Check sheet for the modelled part. Datum: model origin and axes. Units: mm. A direction names the side the tool comes from. Round coordinates to 2 decimals unless told otherwise and drop trailing zeros. Write each loop counter-clockwise with the first axis right and the second up, starting at its lowest first coordinate (ties: lowest second). Pieces come first, ordered by that corner, then holes. Notation, with made-up numbers: M 32,-17 L 50,-17 A24 cw 50,15 Z; hole C 36,34 d5. An arc over 180 degrees is marked long. One line per item, written item: value.
from build123d import *

# Parameters (mm, degrees)
AUFSATZ_LINEAR_AUSTRAGEN1_DEPTH = 20
SKIZZE2_R                       = 3
SCHNITT_LINEAR_AUSTRAGEN1_DEPTH = 20
SKIZZE3_R                       = 5.25
SCHNITT_LINEAR_AUSTRAGEN2_DEPTH = 6.2
SKIZZE4_R                       = 2.3
SCHNITT_LINEAR_AUSTRAGEN3_DEPTH = 10
VERRUNDUNG1_R                   = 2
FASE1_SIZE                      = 0.5


with BuildPart() as part:
    # Skizze1 → Aufsatz-Linear austragen1 (new body)
    with BuildSketch(Plane.XY):
        Polygon((0, -22.130332374), (0, 22.130332374), (7, 22.130332374), (7, 9.485781443), (15.7, 9.485781443), (15.7, -9.485781443), (7, -9.485781443), (7, -22.130332374), align=None)
    extrude(amount=AUFSATZ_LINEAR_AUSTRAGEN1_DEPTH)

    # Skizze2 → Schnitt-Linear austragen1 (cut)
    with BuildSketch(Plane(origin=(15.7, 0, 0), x_dir=(0, 0, -1), z_dir=(1, 0, 0))):
        with Locations((-10, 0)):
            Circle(SKIZZE2_R)
    extrude(amount=-SCHNITT_LINEAR_AUSTRAGEN1_DEPTH, mode=Mode.SUBTRACT)

    # Skizze3 → Schnitt-Linear austragen2 (cut)
    with BuildSketch(Plane.ZY):
        with Locations((10, 0)):
            Circle(SKIZZE3_R)
    extrude(amount=-SCHNITT_LINEAR_AUSTRAGEN2_DEPTH, mode=Mode.SUBTRACT)

    # Skizze4 → Schnitt-Linear austragen3 (cut)
    with BuildSketch(Plane(origin=(7, 0, 0), x_dir=(0, 0, -1), z_dir=(1, 0, 0))):
        with Locations((-10, -15.808056909)):
            Circle(SKIZZE4_R)
        with Locations((-10, 15.808056909)):
            Circle(SKIZZE4_R)
    extrude(amount=-SCHNITT_LINEAR_AUSTRAGEN3_DEPTH, mode=Mode.SUBTRACT)

    # Verrundung1
    verrundung1_edges = [part.edges().sort_by_distance(p)[0] for p in [
        (7, -9.485781443, 10),
        (7, -22.130332374, 10),
        (0, -22.130332374, 10),
        (0, 22.130332374, 10),
        (7, 22.130332374, 10),
        (7, 9.485781443, 10),
        (15.7, 9.485781443, 10),
        (15.7, -9.485781443, 10),
    ]]
    fillet(verrundung1_edges, radius=VERRUNDUNG1_R)

    # Fase1
    fase1_edges = [part.edges().sort_by_distance(p)[0] for p in [
        (15.7, 0, 13),
        (0, 0, 4.75),
        (6.2, 0, 13),
        (0, -15.808056909, 12.3),
        (7, -15.808056909, 12.3),
        (0, 15.808056909, 12.3),
        (7, 15.808056909, 12.3),
        (0, 0, 0),
        (0, 0, 20),
        (11.35, -9.485781443, 0),
        (7, -15.808056909, 0),
        (3.5, -22.130332374, 0),
        (3.5, 22.130332374, 0),
        (7, 15.808056909, 0),
        (11.35, 9.485781443, 0),
        (15.7, 0, 0),
        (0.585786438, -21.544545937, 0),
        (6.414213562, -21.544545937, 0),
        (15.114213562, -8.899995006, 0),
        (15.114213562, 8.899995006, 0),
        (6.414213562, 21.544545937, 0),
        (0.585786438, 21.544545937, 0),
        (3.5, 22.130332374, 20),
        (11.35, -9.485781443, 20),
        (15.7, 0, 20),
        (11.35, 9.485781443, 20),
        (7, 15.808056909, 20),
        (3.5, -22.130332374, 20),
        (7, -15.808056909, 20),
        (0.585786438, -21.544545937, 20),
        (6.414213562, -21.544545937, 20),
        (15.114213562, -8.899995006, 20),
        (15.114213562, 8.899995006, 20),
        (6.414213562, 21.544545937, 20),
        (0.585786438, 21.544545937, 20),
        (7.585786438, -10.071567881, 0),
        (7.585786438, -10.071567881, 20),
        (7.585786438, 10.071567881, 0),
        (7.585786438, 10.071567881, 20),
    ]]
    chamfer(fase1_edges, length=FASE1_SIZE)


solid = part.part
Q1. Draft check along Z on faces 3 (the cylindrical face through (3.542, -15.707, 12.298)), 4 (the cylindrical face through (3.5, 15.9, 12.3)), 5 (the flat face through (6, 0, 20)), 6 (the flat face through (3, 22.13, 10)). Enter one of: pulls with the +Z half, pulls with the -Z half, needs draft (parallel to the pull), parting line crosses it, or undercut.
Completed:
face 3: undercut
face 4: undercut
face 5: pulls with the +Z half
face 6: needs draft
Q2. Access from +Z, -Z, +X, -X, +Y, -Y to the whole of each face (thin tool, end or side, straight path). Record for faces 1 (the cylindrical face through (3.3, 1.6, 15)), 2 (the cylindrical face through (6.4, -21.56, 10.13)).
Completed:
face 1: -X
face 2: +Z, -Z, +X, -Y
Q3. Depth check by flat-ended pin: P1, Ø2, axis at x = 6.5, z = 9, coming from the -Y side; P2, Ø2.5, axis at y = 18, z = 8, coming from the +X side; P3, Ø4, axis at x = 12.5, z = 11.5, coming from the +Y side; P4, Ø11.5, axis at y = -1, z = 10.5, coming from the -X side. Enter the tip coordinate at first touch or a pass-through.
Completed:
P1: y = -22.07
P2: x = 7
P3: y = 9.49
P4: x = 0
Q4. Sectioned sample at C-C on z = 16.25. Enter the section's corners in (x, y).
Completed:
outline: M 0,-20.13 A2 ccw 2,-22.13 L 5,-22.13 A2 ccw 7,-20.13 L 7,-11.49 A2 cw 9,-9.49 L 13.7,-9.49 A2 ccw 15.7,-7.49 L 15.7,7.49 A2 ccw 13.7,9.49 L 9,9.49 A2 cw 7,11.49 L 7,20.13 A2 ccw 5,22.13 L 2,22.13 A2 ccw 0,20.13 Z
Q5. Sectioned sample at D-D on x = 4. Enter the section's corners in (y, z).
Completed:
outline: M -22.13,0.5 L -21.63,0 L 21.63,0 L 22.13,0.5 L 22.13,19.5 L 21.63,20 L -21.63,20 L -22.13,19.5 Z; hole C -15.81,10 d4.6; hole C 0,10 d10.5; hole C 15.81,10 d4.6
Q6. Sectioned sample at A-A on x = 11.5. Enter the section's corners in (y, z).
Completed:
outline: M -9.49,0.5 L -8.99,0 L 8.99,0 L 9.49,0.5 L 9.49,19.5 L 8.99,20 L -8.99,20 L -9.49,19.5 Z; hole C 0,10 d6
Q7. Scan lines: line 1 (Y direction, x = 2.7, z = 10); line 2 (Y direction, x = 12.25, z = 6); line 3 (X direction, y = -12.5, z = 9.25). Record each from-to range of solid material in increasing order. Write a range as [from, to].
Completed:
line 1: [-22.13, -18.11], [-13.51, -5.25], [5.25, 13.51], [18.11, 22.13]
line 2: [-9.49, 9.49]
line 3: [0, 7]
Q8. Sectioned sample at B-B on y = 0. Enter the section's corners in (x, z), and give its area (3 significant figures).
Completed:
outline: M 0,0.5 L 0.5,0 L 15.2,0 L 15.7,0.5 L 15.7,6.5 L 15.2,7 L 6.7,7 L 6.2,6.5 L 6.2,4.75 L 0.5,4.75 L 0,4.25 Z; M 0,15.75 L 0.5,15.25 L 6.2,15.25 L 6.2,13.5 L 6.7,13 L 15.2,13 L 15.7,13.5 L 15.7,19.5 L 15.2,20 L 0.5,20 L 0,19.5 Z
area: 191 mm^2
